from build123d import *

# Parameters (mm, degrees)
ESTRUSIONE_ESTRUSIONE1_DEPTH = 60
SCHIZZO2_R                   = 3.3
TAGLIO_ESTRUSIONE1_DEPTH     = 163.261772004
SCHIZZO3_R                   = 4.5
TAGLIO_ESTRUSIONE2_DEPTH     = 158.032602074


with BuildPart() as part:
    # Schizzo1 → Estrusione-Estrusione1 (new body)
    with BuildSketch(Plane.XY):
        with BuildLine():
            Line((25.014752149, 15.346258777), (56.954134442, 6.506400743))
            add(Edge.make_bspline(
                [(150, 0), (126.370664176, -0.028998352), (94.908093193, -0.705091299), (64.163963919, 4.724970041), (56.954134442, 6.506400743)],
                knots=[0, 0, 0, 0, 0.761803866, 1, 1, 1, 1], degree=3))
            Line((150, 0), (149.992636696, 5.999995482))
            add(Edge.make_bspline(
                [(58.473520543, 12.311445177), (62.126468599, 11.410871011), (69.480954345, 9.870901955), (84.475289112, 7.646971822), (103.507977373, 6.219278985), (126.666543406, 5.867237142), (142.227417194, 5.990465863), (149.992636696, 5.999995482)],
                knots=[0, 0, 0, 0, 0.124885495, 0.24977099, 0.49954198, 0.74931297, 0.99908396, 0.99908396, 0.99908396, 0.99908396], degree=3))
            Line((58.473520543, 12.311445177), (26.615203686, 21.128866742))
            Line((26.615203686, 21.128866742), (25.014752149, 15.346258777))
        make_face()
    extrude(amount=-ESTRUSIONE_ESTRUSIONE1_DEPTH)

    # Schizzo2 → Taglio-Estrusione1 (cut, through all)
    with BuildSketch(Plane(origin=(0, 6, 0), x_dir=(1, 0, 0), z_dir=(0, 1, 0))):
        with Locations(Location((139.992636696, 51, 0), (0, 0, 270))):
            Circle(SCHIZZO2_R)
        with Locations(Location((139.992636696, 9, 0), (0, 0, 270))):
            Circle(SCHIZZO2_R)
    extrude(amount=-TAGLIO_ESTRUSIONE1_DEPTH, mode=Mode.SUBTRACT)

    # Schizzo3 → Taglio-Estrusione2 (cut, through all)
    with BuildSketch(Plane(origin=(7.325457705, 26.467686836, 0), x_dir=(0.9637679941855859, -0.26674192280834413, 0), z_dir=(0.2667419228083441, 0.9637679941855858, 0))):
        with Locations(Location((30.01492693, 51, 0), (0, 0, 180))):
            Circle(SCHIZZO3_R)
        with Locations(Location((30.01492693, 9, 0), (0, 0, 180))):
            Circle(SCHIZZO3_R)
    extrude(amount=-TAGLIO_ESTRUSIONE2_DEPTH, mode=Mode.SUBTRACT)


solid = part.part
Work out the finished part from the listing and answer in its coordinate system (mm). Round coordinates to 2 decimals unless told otherwise and drop trailing zeros. Loops run counter-clockwise (first coordinate to the right, second up) from the corner with the lowest first, then second, coordinate; pieces in that order, holes last. Notation, with made-up numbers: (33, 33) - (88, 33) arc R36 ccw to (88, 67) - close; hole circle Ø8 at (46, 34.25). An arc over 180 degrees is marked (long way). One line per item, written item: value.
Q1. Find section A-A on z = -51. State how many separate pieces and enclosed holes the cut face has, and give its area (3 significant figures).
Check values:
separate pieces: 3
enclosed holes: 0
area: 661 mm2
Q2. Each of these flat-tipped pins is pushed along its axis until it touches: pin 1 Ø8 at (x, z) = (102, -52) entering from -Y; pin 2 Ø7.5 at (x, z) = (139.99, -51) entering from +Y; pin 3 Ø3 at (y, z) = (11.5, -6) entering from -X. Where does it stop, or does it pass through?
Check values:
pin 1: y = 0.34
pin 2: y = 5.98
pin 3: x = 36.02
Q3. The mould has two halves that part along Z. Classify faces 1 (the cylindrical face through (36.404, 15.35, -55.393)), 2 (the flat face through (42.767, 16.658, -29.58)), 3 (the flat face through (87, 7, -60)): +Z half, -Z half, draft (parallel to the pull), parting line (faces both ways), or undercut.
Check values:
face 1: undercut
face 2: draft
face 3: -Z half
Q4. Straight lines are drawn through the part: probe 1 along Z at (x, y) = (142, 5); probe 2 along Y at (x, z) = (144.5, -50); probe 3 along Y at (x, z) = (93, -47). For each, find the intervals that lie inside material, in ascending order.
Check values:
probe 1: -60 to -53.62, -48.38 to -11.62, -6.38 to 0
probe 2: -0.01 to 5.99
probe 3: 1.06 to 7.08
Q5. Find section B-B on x = 53. Give the vertices of the cut face in (y, z), and give its area (3 significant figures).
Check values:
outline: (7.6, -60) - (13.83, -60) - (13.83, 0) - (7.6, 0) - close
area: 374 mm2
